Work out the finished part from the listing and answer in its coordinate system (mm). Give positions to 0.01 mm unless a question says otherwise; leave off trailing zeros. Order: outer loops, then holes, each group sorted by start corner. A loop starts at its lowest first (then second) coordinate and runs counter-clockwise, first axis right, second up.
```python
from build123d import *

# Parameters (mm, degrees)
SKETCH1_R           = 8
SKETCH1_R_2         = 4.15
BOSS_EXTRUDE1_DEPTH = 10
CHAMFER1_SIZE       = 2.6
CHAMFER1_SIZE2      = 1.5011107
FILLET1_R           = 1


with BuildPart() as part:
    # Sketch1 → Boss-Extrude1 (new body)
    with BuildSketch(Plane(origin=(0, 0, 0), x_dir=(1, 0, 0), z_dir=(0, 1, 0))):
        Circle(SKETCH1_R)
        Circle(SKETCH1_R_2, mode=Mode.SUBTRACT)
    extrude(amount=BOSS_EXTRUDE1_DEPTH)

    # Chamfer1
    chamfer1_edges = [part.edges().sort_by_distance(p)[0] for p in [
        (-8, 10, 0),
    ]]
    chamfer1_side = [part.faces().sort_by_distance(p)[0] for p in [
        (-7.77372583, 10, 0),
    ]]
    chamfer(chamfer1_edges, length=CHAMFER1_SIZE, length2=CHAMFER1_SIZE2, reference=chamfer1_side[0])

    # Fillet1
    fillet1_edges = [part.edges().sort_by_distance(p)[0] for p in [
        (-8, 8.4988893, 0),
    ]]
    fillet(fillet1_edges, radius=FILLET1_R)


solid = part.part
```
1. The mould has two halves that part along Z. Classify faces 1 (the face through (7.39, 3.91, 3.06)), 2 (the face through (-0.9, 4.93, 4.05)), 3 (the face through (3.4, 0, 3.4)): pulls with the +Z half, pulls with the -Z half, needs draft (parallel to the pull), parting line crosses it, or undercut.
Findings below:
face 1: parting line crosses it
face 2: undercut
face 3: needs draft
2. The part is cut by section A-A (y = 7.25). Write down the section's boundary in (x, z).
Findings below:
outline: circle Ø16 at (0, 0); hole circle Ø8.3 at (0, 0)
3. Given P1, Ø4, axis at x = -3.5, y = 3.5, coming from the +Z side; P2, Ø1, axis at x = -5, y = 4.5, coming from the -Z side; P3, Ø1, axis at y = 5.5, z = -3.5, coming from the -X side; P4, Ø1.5, axis at x = -1, z = -1, coming from the +Y side, each flat-ended and moving along its own axis, determine where each tip first touches the part or whether it passes through.
Findings below:
P1: stops at z = 7.86
P2: stops at z = -6.61
P3: stops at x = -7.42
P4: passes through
4. Straight lines are drawn through the part: probe 1 along X at (y, z) = (3.25, 0); probe 2 along X at (y, z) = (9, 1.25). For each, find the intervals that lie inside material, in ascending order.
Findings below:
probe 1: x = -8 to -4.15, 4.15 to 8
probe 2: x = -7.02 to -3.96, 3.96 to 7.02
